from build123d import *

# Parameters (mm, degrees)
PAD005_DEPTH           = 170
POCKET001_DEPTH        = 5
LINEARPATTERN_COUNT    = 4
LINEARPATTERN_PITCH    = 50
LINEARPATTERN001_COUNT = 4
LINEARPATTERN001_PITCH = 50
POCKET002_DEPTH        = 5
LINEARPATTERN002_COUNT = 4
LINEARPATTERN002_PITCH = 50
LINEARPATTERN003_COUNT = 4
LINEARPATTERN003_PITCH = 50


with BuildPart() as part:
    # Sketch006 → Pad005 (new body, symmetric)
    with BuildSketch(Plane.YZ):
        Polygon((2, -2), (27, -2), (27, 0), (0, 0), (0, -27), (2, -27), align=None)
    extrude(amount=PAD005_DEPTH, both=True)

    # Sketch007 → Pocket001 (cut)
    with BuildSketch(Plane.XZ):
        with BuildLine():
            ThreePointArc((-10.5, -16), (-13.5, -19), (-10.5, -22))
            Line((-10.5, -22), (10.5, -22))
            ThreePointArc((10.5, -22), (13.5, -19), (10.5, -16))
            Line((-10.5, -16), (10.5, -16))
        make_face()
    pocket001 = extrude(amount=-POCKET001_DEPTH, mode=Mode.SUBTRACT)

    # LinearPattern: Pocket001 ×4
    with Locations(*[(i * LINEARPATTERN_PITCH, 0, 0) for i in range(1, LINEARPATTERN_COUNT)]):
        add(pocket001, mode=Mode.SUBTRACT)

    # LinearPattern001: Pocket001 ×4
    with Locations(*[(-i * LINEARPATTERN001_PITCH, 0, 0) for i in range(1, LINEARPATTERN001_COUNT)]):
        add(pocket001, mode=Mode.SUBTRACT)

    # Sketch008 → Pocket002 (cut)
    with BuildSketch(Plane.XY):
        with BuildLine():
            ThreePointArc((-10.5, 22), (-13.5, 19), (-10.5, 16))
            Line((-10.5, 16), (10.5, 16))
            ThreePointArc((10.5, 16), (13.5, 19), (10.5, 22))
            Line((-10.5, 22), (10.5, 22))
        make_face()
    pocket002 = extrude(amount=-POCKET002_DEPTH, mode=Mode.SUBTRACT)

    # LinearPattern002: Pocket002 ×4
    with Locations(*[(i * LINEARPATTERN002_PITCH, 0, 0) for i in range(1, LINEARPATTERN002_COUNT)]):
        add(pocket002, mode=Mode.SUBTRACT)

    # LinearPattern003: Pocket002 ×4
    with Locations(*[(-i * LINEARPATTERN003_PITCH, 0, 0) for i in range(1, LINEARPATTERN003_COUNT)]):
        add(pocket002, mode=Mode.SUBTRACT)


solid = part.part
Build history of the part. All positions in model axes, mm. A direction names the side the tool comes from. Coordinates: 2 decimals unless noted, no trailing zeros. Write each loop counter-clockwise with the first axis right and the second up, starting at its lowest first coordinate (ties: lowest second). Pieces come first, ordered by that corner, then holes. Notation, with made-up numbers: (75.25, 19.25) -> (109.25, 19.25) arc R29 ccw to (109.25, 47.25) -> close; hole circle Ø1 at (7.5, 79). An arc over 180 degrees is marked (long way). Use CSV: the item, a comma, the result in double quotes. Start each with the question number.
Q1. Cut at B-B, the plane x = -125. List the corners of the cut face in (y, z).
Q2. Cut at A-A, the plane x = 144. List the corners of the cut face in (y, z).
Q3. Flat gauge pin, fed straight in: pin 1 Ø6 at (x, y) = (93.5, 14.5) entering from -Z. Where does the tip first touch, or does it go through?
Q4. Cut at C-C, the plane y = 11.5. List the corners of the cut face in (x, z), then the cut area to 3 significant figures.
Q5. Drill centre lines: probe 1 along Y at (x, z) = (156, -1.25); probe 2 along Y at (x, z) = (23, -12.75); probe 3 along Z at (x, y) = (30, 4.5). Where is each one in solid material? Low to high.
Q6. 3-axis set-ups, long thin cutter, end or side, ignore diameter. For faces 1 (the flat face through (2, 14, -2)), 2 (the flat face through (2, 14, 0)): which of +Z, -Z, +X, -X, +Y, -Y reach the whole face in a straight line?
Q7. Cut at D-D, the plane z = -9.25. List the corners of the cut face in (x, y), then the cut area to 3 significant figures.
Checked values:
1,outline,"(0, -27) -> (2, -27) -> (2, -2) -> (27, -2) -> (27, 0) -> (0, 0) -> close"
2,outline,"(0, -27) -> (2, -27) -> (2, -22) -> (0, -22) -> close; (0, -16) -> (2, -16) -> (2, -2) -> (16, -2) -> (16, 0) -> (0, 0) -> close; (22, -2) -> (27, -2) -> (27, 0) -> (22, 0) -> close"
3,pin 1,"stops at z = -2"
4,outline,"(-170, -2) -> (170, -2) -> (170, 0) -> (-170, 0) -> close"
4,area,"680 mm²"
5,probe 1,"y = 0 to 16, 22 to 27"
5,probe 2,"y = 0 to 2"
5,probe 3,"z = -2 to 0"
6,face 1,"-Z, +X, -X, +Y"
6,face 2,"+Z, +X, -X, +Y, -Y"
7,outline,"(-170, 0) -> (170, 0) -> (170, 2) -> (-170, 2) -> close"
7,area,"680 mm²"
